```python
from build123d import *

# Parameters (mm, degrees)
SKETCH_1_W      = 20
SKETCH_1_H      = 50
SKETCH_1_R      = 2
SKETCH_1_W_2    = 80
SKETCH_1_H_2    = 20
EXTRUDE_1_DEPTH = 3
FILLET_1_R      = 10


with BuildPart() as part:
    # 草图1 → 凸台-拉伸1 (new body)
    # profile 1 of 2: a face of its own
    with BuildSketch(Plane.XY):
        with Locations((0, 35)):
            Rectangle(SKETCH_1_W, SKETCH_1_H)
        with Locations((0, 30)):
            Circle(SKETCH_1_R, mode=Mode.SUBTRACT)
        with Locations((0, 50)):
            Circle(SKETCH_1_R, mode=Mode.SUBTRACT)
    # profile 2 of 2: a face of its own
    with BuildSketch(Plane.XY):
        Rectangle(SKETCH_1_W_2, SKETCH_1_H_2)
        with Locations((30, 0)):
            Circle(SKETCH_1_R, mode=Mode.SUBTRACT)
        with Locations((-30, 0)):
            Circle(SKETCH_1_R, mode=Mode.SUBTRACT)
    extrude(amount=EXTRUDE_1_DEPTH)

    # 圆角1
    fillet_1_edges = [part.edges().sort_by_distance(p)[0] for p in [
        (10, 10, 1.5),
        (-10, 10, 1.5),
    ]]
    fillet(fillet_1_edges, radius=FILLET_1_R)


solid = part.part
```
Verification items for the finished model (mm, model axes). A direction names the side the tool comes from. Coordinates: 2 decimals unless noted, no trailing zeros. Write each loop counter-clockwise with the first axis right and the second up, starting at its lowest first coordinate (ties: lowest second). Pieces come first, ordered by that corner, then holes. Notation, with made-up numbers: (70, 21.25) - (80, 21.25) arc R24 cw to (80, 52.25) - close; hole circle Ø3 at (13, 14.5). An arc over 180 degrees is marked (long way). One line per question, with ' | ' between items. Start each with the question number.
1. Section check D-D (z = 1.05). Enter the section's corners in (x, y).
2. Draft check along X on faces 4 (the cylindrical face through (13.01, 12.85, 1.52)), 5 (the cylindrical face through (0.923, 48.226, 1.479)), 6 (the flat face through (-1, -10, 1)). Enter one of: released by +X, released by -X, zero draft, split by the parting line, or undercut.
3. Section check B-B (x = 0). Enter the section's corners in (y, z).
4. Gauge pin test, flat end, axial feed: P1, Ø0.9, axis at x = 34.5, z = 1.5, coming from the +Y side. Record the tip position at first contact, or that the pin passes through.
5. Access from +Z, -Z, +X, -X, +Y, -Y to the whole of each face (thin tool, end or side, straight path). Record for faces 1 (the flat face through (-1, 18, 3)), 2 (the flat face through (-10, 40, 1)), 3 (the flat face through (30, 10, 1)).
6. Section check A-A (y = 50). Enter the section's corners in (x, z).
7. Section check C-C (y = 0). Enter the section's corners in (x, z), plus the area to 3 significant figures.
8. Material ranges on line 1 along Y through (x, z) = (0, 0.6); line 2 along X through (y, z) = (-1, 2.45); line 3 along X through (y, z) = (20, 2.7), recorded low to high.
Computed values:
1) outline: (-40, -10) - (40, -10) - (40, 10) - (20, 10) arc R10 cw to (10, 20) - (10, 60) - (-10, 60) - (-10, 20) arc R10 cw to (-20, 10) - (-40, 10) - close; hole circle Ø4 at (-30, 0); hole circle Ø4 at (0, 30); hole circle Ø4 at (0, 50); hole circle Ø4 at (30, 0)
2) face 4: released by +X | face 5: undercut | face 6: zero draft
3) outline: (-10, 0) - (28, 0) - (28, 3) - (-10, 3) - close; (32, 0) - (48, 0) - (48, 3) - (32, 3) - close; (52, 0) - (60, 0) - (60, 3) - (52, 3) - close
4) P1: y = 10
5) face 1: +Z, +X, -X, +Y, -Y | face 2: +Z, -Z, -X, +Y | face 3: +Z, -Z, +X, +Y
6) outline: (-10, 0) - (-2, 0) - (-2, 3) - (-10, 3) - close; (2, 0) - (10, 0) - (10, 3) - (2, 3) - close
7) outline: (-40, 0) - (-32, 0) - (-32, 3) - (-40, 3) - close; (-28, 0) - (28, 0) - (28, 3) - (-28, 3) - close; (32, 0) - (40, 0) - (40, 3) - (32, 3) - close | area: 216 mm²
8) line 1: -10 to 28, 32 to 48, 52 to 60 | line 2: -40 to -31.73, -28.27 to 28.27, 31.73 to 40 | line 3: -10 to 10
